from build123d import *

# Parameters (mm, degrees)
ESQUISSE1_W             = 20
ESQUISSE1_H             = 20
BOSS_EXTRU_1_DEPTH      = 50
ESQUISSE2_W             = 22.5
ESQUISSE2_H             = 22.5
BOSS_EXTRU_2_DEPTH      = 50
ESQUISSE5_W             = 22.5
ESQUISSE5_H             = 22.5
ESQUISSE4_W             = 20
ESQUISSE4_H             = 20
ENL_V_MAT_EXTRU_1_REACH = 24.5
ESQUISSE6_R             = 2.25
ENL_V_MAT_EXTRU_2_REACH = 23.25
ESQUISSE7_R             = 2.25


with BuildPart() as part:
    # Esquisse1 → Boss.-Extru.1 (new body)
    with BuildSketch(Plane.XY):
        with Locations((-32.865009747, 8)):
            Rectangle(ESQUISSE1_W, ESQUISSE1_H)
    extrude(amount=BOSS_EXTRU_1_DEPTH)



with BuildPart() as body_2:
    # Esquisse2 → Boss.-Extru.2 (new body)
    with BuildSketch(Plane(origin=(0, 0, -92), x_dir=(-1, 0, 0), z_dir=(0, 0, -1))):
        with Locations((32.865009747, 8)):
            Rectangle(ESQUISSE2_W, ESQUISSE2_H)
    extrude(amount=-BOSS_EXTRU_2_DEPTH)


with BuildPart() as part_1:
    add(part.part)

    add(body_2.part)  # Lissage1 merges body 2
    # Esquisse5 → Lissage1 section 0
    with BuildSketch(Plane.XY.offset(-42)):
        with Locations((-32.865009747, 8)):
            Rectangle(ESQUISSE5_W, ESQUISSE5_H)
    # Esquisse4 → Lissage1 section 1
    with BuildSketch(Plane(origin=(0, 0, 0), x_dir=(-1, 0, 0), z_dir=(0, 0, -1))):
        with Locations((32.865009747, 8)):
            Rectangle(ESQUISSE4_W, ESQUISSE4_H)
    loft()

    # Esquisse6 → Enlèv. mat.-Extru.1 (cut, up to next)
    with BuildSketch(Plane(origin=(0, 19.25, 0), x_dir=(1, 0, 0), z_dir=(0, 1, 0)), mode=Mode.PRIVATE) as enl_v_mat_extru_1_sk1:
        with Locations((-32.865009747, 82)):
            Circle(ESQUISSE6_R)
    enl_v_mat_extru_1_tool1 = extrude(enl_v_mat_extru_1_sk1.sketch, amount=-ENL_V_MAT_EXTRU_1_REACH, mode=Mode.PRIVATE) & part_1.part
    add(enl_v_mat_extru_1_tool1.solids().sort_by_distance((-32.86501, 19.25, -82))[0], mode=Mode.SUBTRACT)

    # Esquisse7 → Enlèv. mat.-Extru.2 (cut, up to next)
    with BuildSketch(Plane.XZ.offset(2), mode=Mode.PRIVATE) as enl_v_mat_extru_2_sk1:
        with Locations((-32.865009747, 40)):
            Circle(ESQUISSE7_R)
    enl_v_mat_extru_2_tool1 = extrude(enl_v_mat_extru_2_sk1.sketch, amount=-ENL_V_MAT_EXTRU_2_REACH, mode=Mode.PRIVATE) & part_1.part
    add(enl_v_mat_extru_2_tool1.solids().sort_by_distance((-32.86501, -2, 40))[0], mode=Mode.SUBTRACT)


solid = part_1.part
Build history of the part. All positions in model axes, mm. A direction names the side the tool comes from. Round coordinates to 2 decimals unless told otherwise and drop trailing zeros. Write each loop counter-clockwise with the first axis right and the second up, starting at its lowest first coordinate (ties: lowest second). Pieces come first, ordered by that corner, then holes. Notation, with made-up numbers: (32, 58.25) - (79, 58.25) arc R16 cw to (79, 69.25) - close; hole circle Ø4 at (-3, 18). An arc over 180 degrees is marked (long way). Use CSV: the item, a comma, the result in double quotes.
(1) Band-saw the part on B-B (z = -82). Write the cut outline in (x, y) (3 decimals).
Response:
outline,"(-44.115, -3.25) - (-35.115, -3.25) - (-35.115, 19.25) - (-44.115, 19.25) - close; (-30.615, -3.25) - (-21.615, -3.25) - (-21.615, 19.25) - (-30.615, 19.25) - close"
(2) Wall check: line 1 (Z direction, x = -33, y = 2.25); line 2 (Z direction, x = -31.5, y = 0); line 3 (X direction, y = 5.75, z = -82) (3 decimals). Give the ranges that are in metal, low to high.
Response:
line 1,"-92 to -84.25, -79.75 to 37.75, 42.25 to 50"
line 2,"-92 to -83.79, -80.21 to 38.21, 41.79 to 50"
line 3,"-44.115 to -35.115, -30.615 to -21.615"
(3) 3-axis set-ups, long thin cutter, end or side, ignore diameter. For faces 4 (the flat face through (-42.865, 8, 25)), 5 (the flat face through (-33, -2, 25)), 6 (the flat face through (-33, -3.25, -67)), 7 (the flat face through (-33, 18, 25)): which of +Z, -Z, +X, -X, +Y, -Y reach the whole face in a straight line?
Response:
face 4,"+Z, -X, +Y, -Y"
face 5,"+Z, +X, -X, -Y"
face 6,"+Z, -Z, +X, -X, -Y"
face 7,"+Z, +X, -X, +Y"
(4) Mould opens along Z. For faces 1 (the flat face through (-33, 8, 50)), 2 (the flat face through (-22.865, 8, 25)), 3 (the cylindrical face through (-31.66, 7.86, 41.9)) say: pulls with the +Z half, pulls with the -Z half, needs draft (parallel to the pull), parting line crosses it, or undercut.
Response:
face 1,"pulls with the +Z half"
face 2,"needs draft"
face 3,"undercut"
(5) Band-saw the part on C-C (y = 6). Give the number of separate pieces and of enclosed holes in the cut face, plus the area to 3 significant figures.
Response:
separate pieces,"1"
enclosed holes,"2"
area,"2,990 mm²"
(6) Band-saw the part on A-A (z = 40). Write the cut outline in (x, y) (3 decimals), plus the area to 3 significant figures.
Response:
outline,"(-42.865, -2) - (-35.115, -2) - (-35.115, 18) - (-42.865, 18) - close; (-30.615, -2) - (-22.865, -2) - (-22.865, 18) - (-30.615, 18) - close"
area,"310 mm²"
(7) Pin check, flat tips, straight feed: P1, Ø6, axis at x = -32.87, z = -82, coming from the -Y side; P2, Ø1.5, axis at y = 0, z = -16.5, coming from the -X side; P3, Ø12, axis at y = 3, z = 8.5, coming from the +X side (3 decimals); P4, Ø4, axis at x = -32.87, z = 40, coming from the +Y side. Stop position of each tip, or through.
Response:
P1,"y = -3.25"
P2,"x = -43.38"
P3,"x = -22.865"
P4,"through"
